from build123d import *

# Parameters (mm, degrees)
SKETCH1_W           = 95.5
SKETCH1_H           = 44
BOSS_EXTRUDE1_DEPTH = 5
SKETCH2_R           = 1.5
CUT_EXTRUDE1_DEPTH  = 6
SKETCH3_W           = 20
SKETCH3_H           = 44
SKETCH3_R           = 2
BOSS_EXTRUDE2_DEPTH = 5


with BuildPart() as part:
    # Sketch1 → Boss-Extrude1 (new body)
    with BuildSketch(Plane(origin=(0, 0, 0), x_dir=(1, 0, 0), z_dir=(0, 1, 0))):
        Rectangle(SKETCH1_W, SKETCH1_H)
    extrude(amount=BOSS_EXTRUDE1_DEPTH)

    # Sketch2 → Cut-Extrude1 (cut, through all)
    with BuildSketch(Plane(origin=(0, 5, 0), x_dir=(1, 0, 0), z_dir=(0, 1, 0))):
        with Locations((-43.75, 18)):
            Circle(SKETCH2_R)
        with Locations((-20.25, 18)):
            Circle(SKETCH2_R)
        with Locations((3.25, 18)):
            Circle(SKETCH2_R)
        with Locations((26.75, 18)):
            Circle(SKETCH2_R)
    extrude(amount=-CUT_EXTRUDE1_DEPTH, mode=Mode.SUBTRACT)

    # Sketch3 → Boss-Extrude2 (add)
    with BuildSketch(Plane(origin=(0, 5, 0), x_dir=(1, 0, 0), z_dir=(0, 1, 0))):
        with Locations((57.75, 0)):
            Rectangle(SKETCH3_W, SKETCH3_H)
        with Locations((57.75, 12)):
            Circle(SKETCH3_R, mode=Mode.SUBTRACT)
        with Locations((57.75, -12)):
            Circle(SKETCH3_R, mode=Mode.SUBTRACT)
    extrude(amount=-BOSS_EXTRUDE2_DEPTH)


solid = part.part
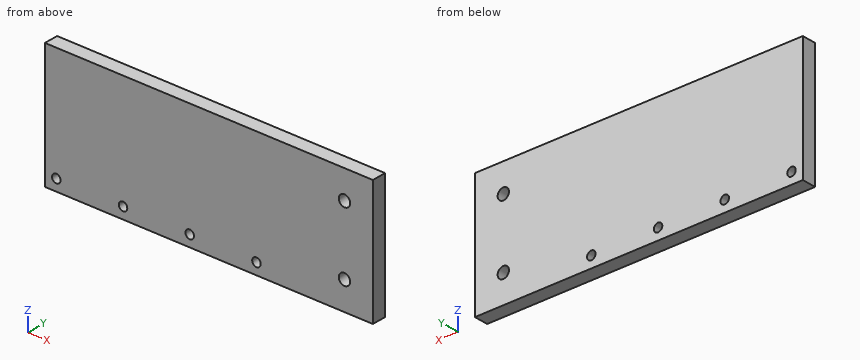
Can you work these out from the model? Positions are in its coordinate system, mm. Give positions to 0.01 mm unless a question says otherwise; leave off trailing zeros. Loops run counter-clockwise (first coordinate to the right, second up) from the corner with the lowest first, then second, coordinate; pieces in that order, holes last. Notation, with made-up numbers: M -5,57.25 L 42,57.25 A26 ccw 42,88.25 Z; hole C 67,49.25 d1. An arc over 180 degrees is marked long. One line per item, written item: value.
1) I'm going to push a flat-ended pin straight in: pin 1 (2.5 mm diameter, centred on x = -20.25, z = -18, fed in from +Y). Where does the tip first touch, or does it pass through?
Geometry check:
pin 1: passes through
2) Imagine slicing it at D-D on x = 26.75. Write out the boundary of the cut face in (y, z).
Geometry check:
outline: M 0,-22 L 5,-22 L 5,-19.5 L 0,-19.5 Z; M 0,-16.5 L 5,-16.5 L 5,22 L 0,22 Z
3) Imagine slicing it at A-A on z = -12. Write out the boundary of the cut face in (x, y), and give its area (4 significant figures).
Geometry check:
outline: M -47.75,0 L 55.75,0 L 55.75,5 L -47.75,5 Z; M 59.75,0 L 67.75,0 L 67.75,5 L 59.75,5 Z
area: 557.5 mm²
4) Please list where these lines run through material, in increasing order: line 1 (Z direction, x = 57.75, y = 3.6); line 2 (X direction, y = 1.3, z = -18); line 3 (Z direction, x = 3.25, y = 1.05).
Geometry check:
line 1: z = -22 to -14, -10 to 10, 14 to 22
line 2: x = -47.75 to -45.25, -42.25 to -21.75, -18.75 to 1.75, 4.75 to 25.25, 28.25 to 67.75
line 3: z = -22 to -19.5, -16.5 to 22
5) Imagine slicing it at B-B on x = 57.75. Write out the boundary of the cut face in (y, z), and give its area (3 significant figures).
Geometry check:
outline: M 0,-22 L 5,-22 L 5,-14 L 0,-14 Z; M 0,-10 L 5,-10 L 5,10 L 0,10 Z; M 0,14 L 5,14 L 5,22 L 0,22 Z
area: 180 mm²
6) Imagine slicing it at C-C on z = -18. Write out the boundary of the cut face in (x, y), and give its area (4 significant figures).
Geometry check:
outline: M -47.75,0 L -45.25,0 L -45.25,5 L -47.75,5 Z; M -42.25,0 L -21.75,0 L -21.75,5 L -42.25,5 Z; M -18.75,0 L 1.75,0 L 1.75,5 L -18.75,5 Z; M 4.75,0 L 25.25,0 L 25.25,5 L 4.75,5 Z; M 28.25,0 L 67.75,0 L 67.75,5 L 28.25,5 Z
area: 517.5 mm²
